```python
from build123d import *

# Parameters (mm, degrees)
SKETCH1_W           = 200
SKETCH1_H           = 100
BOSS_EXTRUDE2_DEPTH = 3.18
SKETCH2_R           = 1.55
SKETCH2_W           = 3.18
SKETCH2_H           = 40.125
CUT_EXTRUDE1_DEPTH  = 4.18


with BuildPart() as part:
    # Sketch1 → Boss-Extrude2 (new body)
    with BuildSketch(Plane.XY):
        Rectangle(SKETCH1_W, SKETCH1_H)
    extrude(amount=BOSS_EXTRUDE2_DEPTH)

    # Sketch2 → Cut-Extrude1 (cut, through all)
    with BuildSketch(Plane.XY.offset(3.18)):
        with Locations((-98, 0)):
            Circle(SKETCH2_R)
        Polygon((-10, 50), (-10, 46.82), (-1.5, 46.82), (-1.5, 42.82), (-3.25, 42.82), (-3.25, 39.82), (-1.5, 39.82), (-1.5, 37), (1.5, 37), (1.5, 39.82), (3.25, 39.82), (3.25, 42.82), (1.5, 42.82), (1.5, 46.82), (10, 46.82), (10, 50), align=None)
        with Locations((-98.41, 29.9375)):
            Rectangle(SKETCH2_W, SKETCH2_H)
        with Locations((-98.41, -29.9375)):
            Rectangle(SKETCH2_W, SKETCH2_H)
    cut_extrude1 = extrude(amount=-CUT_EXTRUDE1_DEPTH, mode=Mode.SUBTRACT)

    # Mirror1: Cut-Extrude1 across plane
    add(cut_extrude1.mirror(Plane.ZX), mode=Mode.SUBTRACT)

    # Mirror2: Cut-Extrude1 across plane
    add(cut_extrude1.mirror(Plane(origin=(0, 0, 0), x_dir=(0, 0, 1), z_dir=(1, 0, 0))), mode=Mode.SUBTRACT)


solid = part.part
```
Work out the finished part from the listing and answer in its coordinate system (mm). Round coordinates to 2 decimals unless told otherwise and drop trailing zeros. Order: outer loops, then holes, each group sorted by start corner. A loop starts at its lowest first (then second) coordinate and runs counter-clockwise, first axis right, second up.
Q1. Given pin 1 Ø0.9 at (x, z) = (3, 2) entering from +Y; pin 2 Ø1 at (y, z) = (-27, 1) entering from +X; pin 3 Ø2.5 at (x, y) = (-98, 0) entering from +Z; pin 4 Ø1.5 at (x, z) = (-0.5, 2) entering from -Y, each flat-ended and moving along its own axis, determine where each tip first touches the part or whether it passes through.
Solution:
pin 1: stops at y = 46.82
pin 2: stops at x = 96.82
pin 3: passes through
pin 4: stops at y = -37
Q2. A cutting plane is placed at A-A, the plane z = 1.55. Count the separate pieces of the cut face and the enclosed holes in it, then the cut area to 3 significant figures.
Solution:
separate pieces: 1
enclosed holes: 2
area: 19,300 mm2
Q3. Find the intervals of material crossed by line 1 along Y through (x, z) = (-98, 1.85) (3 decimals); line 2 along X through (y, z) = (-1, 1.5); line 3 along X through (y, z) = (22, 1.5), in increasing order.
Solution:
line 1: y = -9.875 to -1.55, 1.55 to 9.875
line 2: x = -100 to -99.18, -96.82 to 96.82, 99.18 to 100
line 3: x = -96.82 to 96.82
Q4. A cutting plane is placed at B-B, the plane y = 27. Determine the outline of the cut face in (x, z).
Solution:
outline: (-96.82, 0) - (96.82, 0) - (96.82, 3.18) - (-96.82, 3.18) - close
